Work out the finished part from the listing and answer in its coordinate system (mm). A direction names the side the tool comes from. Round coordinates to 2 decimals unless told otherwise and drop trailing zeros. Order: outer loops, then holes, each group sorted by start corner. A loop starts at its lowest first (then second) coordinate and runs counter-clockwise, first axis right, second up. Notation, with made-up numbers: (24, 86) - (72, 86) arc R25 cw to (72, 114) - close; hole circle Ø5 at (27, 1). An arc over 180 degrees is marked (long way). Use one line per item in the form item = value. Start each with the question number.
Q1. Which of the six approach directions +Z, -Z, +X, -X, +Y, -Y give full straight-line access (tool end or side, diameter ignored) to faces 1 (the cylindrical face through (-9.76, 18.99, -2.17)), 2 (the flat face through (0.1, 5, -3.4)), 3 (the cylindrical face through (2.703, 9.902, 8.584)), 4 (the flat face through (-8.1, 0, -0.8)), 5 (the cylindrical face through (4.837, 17.465, 6.309))?
Q2. Find the intervals of material crossed by line 1 (X direction, y = 1.85, z = 0); line 2 (X direction, y = 11.75, z = 0); line 3 (Y direction, x = -2, z = -6), in increasing order. Write a range as [from, to].
Q3. Given P1, Ø4, axis at x = 8, y = 10.5, coming from the -Z side; P2, Ø9.5, axis at x = 0, z = 0, coming from the -Y side; P3, Ø1.5, axis at y = 10, z = 6, coming from the -X side, each flat-ended and moving along its own axis, determine where each tip first touches the part or whether it passes through.
Q4. The part is cut by section D-D on y = 16.5. Determine the outline of the cut face in (x, z).
Q5. The part is cut by section C-C on y = 11.75. Determine the outline of the cut face in (x, z), plus the area to 3 significant figures.
Q6. For a pull along X with two mould halves and no side action, classify faces 6 (the flat face through (-8.1, 20, -0.8)), 7 (the flat face through (-0.1, 15, -3.4)), 8 (the cylindrical face through (-9.76, 1.01, -2.17)) as +X half, -X half, draft (parallel to the pull), parting line (faces both ways), or undercut.
from build123d import *

# Parameters (mm, degrees)
SKETCH_1_R          = 8
SKETCH_1_R_2        = 3
EXTRUDE_1_DEPTH     = 20
EXTRUDE_START       = -20
SKETCH_2_R          = 9
SKETCH_2_R_2        = 3
EXTRUDE_2_DEPTH     = 20
EXTRUDE_START_2     = -2
SKETCH_3_R          = 10
SKETCH_3_R_2        = 9
EXTRUDE_3_DEPTH     = 2
FILLET_1_R          = 1
FILLET_2_R          = 1
SKETCH_4_R          = 7.95
CUT_EXTRUDE_1_DEPTH = 5
CUT_EXTRUDE_START   = -5
SKETCH_5_R          = 7.95
CUT_EXTRUDE_2_DEPTH = 5


with BuildPart() as part:
    # 草图1 → 凸台-拉伸1 (new body)
    with BuildSketch(Plane(origin=(0, 0, 0), x_dir=(1, 0, 0), z_dir=(0, 1, 0))):
        with Locations(Location((0, 0, 0), (0, 0, 270))):
            Circle(SKETCH_1_R)
        with Locations(Location((0, 0, 0), (0, 0, 270))):
            Circle(SKETCH_1_R_2, mode=Mode.SUBTRACT)
    extrude(amount=EXTRUDE_1_DEPTH)

    # 草图2 → 凸台-拉伸2 (add)
    with BuildSketch(Plane(origin=(0, 20, 0), x_dir=(1, 0, 0), z_dir=(0, 1, 0)).offset(EXTRUDE_START)):
        with Locations(Location((0, 0, 0), (0, 0, 270))):
            Circle(SKETCH_2_R)
        with Locations(Location((0, 0, 0), (0, 0, 270))):
            Circle(SKETCH_2_R_2, mode=Mode.SUBTRACT)
    extrude(amount=EXTRUDE_2_DEPTH)

    # 草图3 → 凸台-拉伸3 (add)
    with BuildSketch(Plane(origin=(0, 20, 0), x_dir=(1, 0, 0), z_dir=(0, 1, 0)).offset(EXTRUDE_START_2)):
        with Locations(Location((0, 0, 0), (0, 0, 270))):
            Circle(SKETCH_3_R)
        with Locations(Location((0, 0, 0), (0, 0, 270))):
            Circle(SKETCH_3_R_2, mode=Mode.SUBTRACT)
    extrude_3 = extrude(amount=EXTRUDE_3_DEPTH)

    # 镜向1: 凸台-拉伸3 across plane
    add(extrude_3.mirror(Plane(origin=(0, 10, 0), x_dir=(0, 0, 1), z_dir=(0, -1, 0))))

    # 圆角1
    fillet_1_edges = [part.edges().sort_by_distance(p)[0] for p in [
        (0, 18, -9),
    ]]
    fillet(fillet_1_edges, radius=FILLET_1_R - 0.0001)  # a hair under: the kernel refuses the full size

    # 圆角2
    fillet_2_edges = [part.edges().sort_by_distance(p)[0] for p in [
        (0, 2, -9),
    ]]
    fillet(fillet_2_edges, radius=FILLET_2_R - 0.0001)  # a hair under: the kernel refuses the full size

    # 草图4 → 切除-拉伸1 (cut)
    with BuildSketch(Plane.XZ):
        with Locations(Location((0, 0, 0), (0, 0, 270))):
            Circle(SKETCH_4_R)
    extrude(amount=-CUT_EXTRUDE_1_DEPTH, mode=Mode.SUBTRACT)

    # 草图5 → 切除-拉伸2 (cut)
    with BuildSketch(Plane(origin=(0, 20, 0), x_dir=(1, 0, 0), z_dir=(0, 1, 0)).offset(CUT_EXTRUDE_START)):
        with Locations(Location((0, 0, 0), (0, 0, 90))):
            Circle(SKETCH_5_R)
    extrude(amount=CUT_EXTRUDE_2_DEPTH, mode=Mode.SUBTRACT)


solid = part.part
Found:
q1.face_1 = +Y, -Y
q1.face_2 = -Y
q1.face_3 = none
q1.face_4 = +Z, -Z, +X, -X, -Y
q1.face_5 = +Y
q2.line_1 = [-10, -7.95], [7.95, 10]
q2.line_2 = [-9, -3], [3, 9]
q2.line_3 = [5, 15]
q3.P1 = -6.71
q3.P2 = 5
q3.P3 = -7.31
q4.outline = circle Ø18 at (0, 0); hole circle Ø15.9 at (0, 0)
q5.outline = circle Ø18 at (0, 0); hole circle Ø6 at (0, 0)
q5.area = 226 mm²
q6.face_6 = draft
q6.face_7 = undercut
q6.face_8 = parting line
